Autodesk Inventor part; units mm, degrees
ref_plane "YZ Plane" through (0, 0, 0) normal (1, 0, 0) x (0, 1, 0)
ref_plane "XZ Plane" through (0, 0, 0) normal (0, 1, 0) x (-1, 0, 0)
ref_plane "XY Plane" through (0, 0, 0) normal (0, 0, 1) x (1, 0, 0)
sketch "Sketch1" plane through (0, 0, 0) normal (0, 0, 1) x (1, 0, 0)
  line L0 (-90, 100) -> (90, 100)
  line L1 (90, 100) -> (90, -100)
  line L2 (90, -100) -> (-90, -100)
  line L3 (-90, -100) -> (-90, 100)
  line L4 (-90, 100) -> (90, -100) construction
  line L5 (90, 100) -> (-90, -100) construction
  point P0 (0, 0)
  dimension "d0" = 180
  dimension "d1" = 200
extrude "Plate1" add sketch "Sketch1" along normal blind 4
sketch "Sketch2" plane through (0, 0, 0) normal (0, 0, 1) x (1, 0, 0)
  circle A0 centre (0, 0) radius 45
  dimension "d3" = 90
extrude "Extrusion1" cut sketch "Sketch2" along normal blind 10
equation "\"d2\" = Thickness"
equation "\"BendRadius\" = Thickness"
equation "\"BendReliefWidth\" = Thickness"
equation "\"BendReliefDepth\" = 0.5 * Thickness"
equation "\"CornerReliefSize\" = 4 * Thickness"
equation "\"MinimumRemnant\" = 2 * Thickness"
equation "\"TransitionRadius\" = BendRadius"
equation "\"JacobiRadiusSize\" = BendRadius"
equation "\"GapSize\" = Thickness"
equation "\"Конус_Угол_продольный\" = 52.4deg"
equation "\"Конус_Угол_поперечный\" = 52deg"
properties part number "MSC 111 cone IN bottom" material "Stainless Steel"
Source: CAD feature listing. Evaluate the final solid. Frame: model axes, mm. Give positions to 0.01 mm unless a question says otherwise; leave off trailing zeros. Write each loop counter-clockwise with the first axis right and the second up, starting at its lowest first coordinate (ties: lowest second). Pieces come first, ordered by that corner, then holes.
1. Section query B-B (x = 0). Return the cut outline in (y, z).
2. Material intervals for line 1 along X through (y, z) = (0, 2.1); line 2 along Y through (x, z) = (0, 2.9); line 3 along X through (y, z) = (12, 0.25), sorted ascending.
3. Pull-direction query (X, two-part tool) for faces 1 (the face through (-1, 46, 0)), 2 (the face through (20.765, 39.923, 1.972)); classes: +X half, -X half, draft (parallel to the pull), parting line (faces both ways), or undercut.
4. Section query A-A (y = 0). Return the cut outline in (x, z), then the cut area to 3 significant figures.
5. Section query C-C (z = 2.95). Return the cut outline in (x, y), then the cut area to 3 significant figures.
Output values:
1. outline: (-100, 0) - (-45, 0) - (-45, 4) - (-100, 4) - close; (45, 0) - (100, 0) - (100, 4) - (45, 4) - close
2. line 1: x = -90 to -45, 45 to 90
2. line 2: y = -100 to -45, 45 to 100
2. line 3: x = -90 to -43.37, 43.37 to 90
3. face 1: draft
3. face 2: undercut
4. outline: (-90, 0) - (-45, 0) - (-45, 4) - (-90, 4) - close; (45, 0) - (90, 0) - (90, 4) - (45, 4) - close
4. area: 360 mm2
5. outline: (-90, -100) - (90, -100) - (90, 100) - (-90, 100) - close; hole circle Ø90 at (0, 0)
5. area: 29,600 mm2
